```python
from build123d import *

# Parameters (mm, degrees)
F0_R     = 2
F1_DEPTH = 24
F2_R     = 5
F2_R_2   = 2
F3_DEPTH = 3


# Not quite as in the source:
# - a fillet or chamfer that OpenCascade refuses, or shapes differently, is made with other operations: its cross-section is extruded or revolved along the edge and cut away or added


with BuildPart() as f1:
    # F0 (on Front) → F1 (new body)
    with BuildSketch(Plane.XZ):
        Circle(F0_R)
    extrude(amount=F1_DEPTH)

    # F2 (on face) → F3 (join)
    with BuildSketch(Plane.XZ.offset(24)):
        Circle(F2_R)
        Circle(F2_R_2, mode=Mode.SUBTRACT)
        Circle(F2_R_2)
    extrude(amount=F3_DEPTH)

    # F4: fillet of radius 5 on 1 edges, made by hand

    # F4_s1 → F4_t2 (revolve, cut)
    with BuildSketch(Plane.XY):
        with BuildLine():
            ThreePointArc((5, -24), (3.1560370926, -26.1833001327), (0.417424305, -27))
            Line((0.417424305, -27), (5, -27))
            Line((5, -27), (5, -24))
        make_face()
    revolve(axis=Axis((0, -27, 0), (0, -1, 0)), mode=Mode.SUBTRACT)


solid = f1.part
```
Model file for the job. Use its own axes, mm. A direction names the side the tool comes from. Coordinates: 2 decimals unless noted, no trailing zeros. Write each loop counter-clockwise with the first axis right and the second up, starting at its lowest first coordinate (ties: lowest second). Pieces come first, ordered by that corner, then holes. Notation, with made-up numbers: (40.25, -4) - (87.25, -4) arc R14 cw to (87.25, 0) - close; hole circle Ø8 at (35.25, 51). An arc over 180 degrees is marked (long way). One line per item, written item: value. Start each with the question number.
1. Slice it at A-A (y = -11.75). Write the cut outline in (x, z), plus the area to 3 significant figures.
2. Tool access for faces 1 (the cylindrical face through (0, -12, -2)), 2 (the flat face through (0, 0, 0)): list every direction of +Z, -Z, +X, -X, +Y, -Y with a clear straight run to the whole face (end or side of a thin tool).
3. Flat gauge pins, fed straight in: pin 1 (6 mm diameter, centred on y = -15, z = -3.5, fed in from +X); pin 2 (4 mm diameter, centred on x = 3, z = 3, fed in from +Y); pin 3 (1 mm diameter, centred on x = 0, y = -6, fed in from +Z). Where does each tip first touch, or does it go through?
4. Probe line 1 (Z direction, x = 0, y = -11.5); line 2 (Y direction, x = -0.25, z = 0.5); line 3 (Y direction, x = -1.5, z = -4.25). List the from-to ranges inside material, lowest first. Write a range as from..to.
Answers below:
1. outline: circle Ø4 at (0, 0)
1. area: 12.6 mm^2
2. face 1: +Y
2. face 2: +Z, -Z, +X, -X, +Y
3. pin 1: stops at x = 1.94
3. pin 2: stops at y = -24
3. pin 3: stops at z = 2
4. line 1: z = -2..2
4. line 2: y = -27..0
4. line 3: y = -24.88..-24
